The listing builds one solid part. Answer for the finished solid, in the listing's coordinates (mm). Face numbers are marked on the shaded views. A direction names the side the tool comes from. Round coordinates to 2 decimals unless told otherwise and drop trailing zeros. Order: outer loops, then holes, each group sorted by start corner. A loop starts at its lowest first (then second) coordinate and runs counter-clockwise, first axis right, second up. Notation, with made-up numbers: M 78.5,-38 L 122.5,-38 A19 cw 122.5,-3 Z; hole C -12,13 d2. An arc over 180 degrees is marked long. Put each result on its own line as item: value. Start each with the question number.
1. The part is cut by section B-B (z = 8). Give the vertices of the cut face in (x, y), then the cut area to 3 significant figures.
2. The part is cut by section C-C (z = 4.5). Give the vertices of the cut face in (x, y), then the cut area to 3 significant figures.
3. Which of the six approach directions +Z, -Z, +X, -X, +Y, -Y give full straight-line access (tool end or side, diameter ignored) to the marked faces 1 and 2?
4. Consider line 1 (Z direction, x = -0.7, y = 10); line 2 (X direction, y = 5, z = -7.75); line 3 (Y direction, x = 41, z = -1.5). Determine where each line is inside the solid, lowest interval first.
5. Each of these flat-tipped pins is pushed along its axis until it touches: pin 1 Ø1 at (x, z) = (41, 11.5) entering from +Y; pin 2 Ø12 at (x, z) = (35, 0) entering from -Y; pin 3 Ø3 at (x, z) = (38, -10) entering from +Y. Where does it stop, or does it pass through?
6. The part is cut by section A-A (y = 11.5). Give the vertices of the cut face in (x, z).
7. The part is cut by section D-D (x = 47.5). Give the vertices of the cut face in (y, z).
from build123d import *

# Parameters (mm, degrees)
SM_BASE_FLANGE_1_DEPTH = 15
SKETCH_6_R             = 2.5
CUT_EXTRUDE_664_DEPTH  = 10
SKETCH_7_R             = 6.5
CUT_EXTRUDE_2_DEPTH    = 10


# Sheet-metal steps are written as plain solids
with BuildPart() as part:
    # Sketch 1 → Базовая кромка1 (new, symmetric)
    with BuildSketch(Plane.XY):
        with BuildLine():
            Line((0, 20), (0, 1.089813792))
            ThreePointArc((0, 1.089813792), (0.286474508, 0.208135914), (1.036474508, -0.336770982))
            Line((1.036474508, -0.336770982), (52.308108396, -16.995934691))
            Line((52.308108396, -16.995934691), (51.844582905, -18.422519465))
            Line((51.844582905, -18.422519465), (0.572949017, -1.763355757))
            ThreePointArc((0.572949017, -1.763355757), (-0.927050983, -0.673541965), (-1.5, 1.089813792))
            Line((-1.5, 1.089813792), (-1.5, 20))
            Line((-1.5, 20), (0, 20))
        make_face()
    extrude(amount=SM_BASE_FLANGE_1_DEPTH, both=True)

    # Эскиз6 → Cut-Extrude 664 (cut)
    with BuildSketch(Plane(origin=(0, 0, 0), x_dir=(0, 0, -1), z_dir=(1, 0, 0))):
        with Locations(Location((-8, 10, 0), (0, 0, 90))):
            Circle(SKETCH_6_R)
        with Locations(Location((8, 10, 0), (0, 0, 90))):
            Circle(SKETCH_6_R)
    extrude(amount=-CUT_EXTRUDE_664_DEPTH, mode=Mode.SUBTRACT)

    # Эскиз7 → Вырез-Вытянуть2 (cut)
    with BuildSketch(Plane(origin=(0, 0, 0), x_dir=(0.9510565162951546, -0.3090169943749447, 0), z_dir=(0.3090169943749447, 0.9510565162951546, 0))):
        with Locations(Location((30, 0, 0), (0, 0, 180))):
            Circle(SKETCH_7_R)
    extrude(amount=-CUT_EXTRUDE_2_DEPTH, mode=Mode.SUBTRACT)


solid = part.part
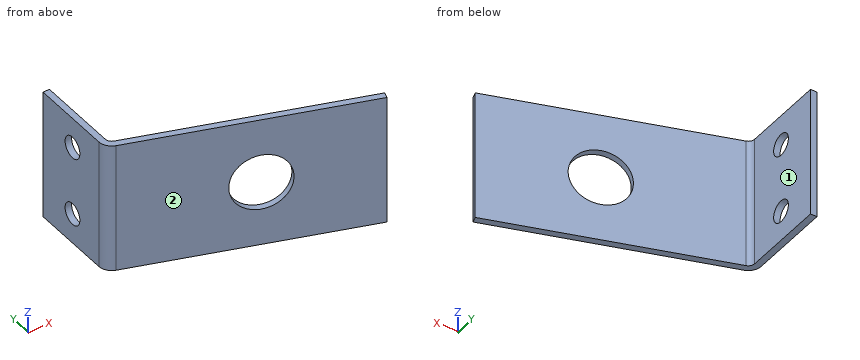
Resolved:
1. outline: M -1.5,1.09 A3 ccw 0.57,-1.76 L 51.84,-18.42 L 52.31,-17 L 1.04,-0.34 A1.5 cw 0,1.09 L 0,7.5 L -1.5,7.5 Z; M -1.5,12.5 L 0,12.5 L 0,20 L -1.5,20 Z
1. area: 106 mm2
2. outline: M -1.5,1.09 A3 ccw 0.57,-1.76 L 23.61,-9.25 L 24.07,-7.82 L 1.04,-0.34 A1.5 cw 0,1.09 L 0,20 L -1.5,20 Z; M 32.53,-12.15 L 51.84,-18.42 L 52.31,-17 L 32.99,-10.72 Z
2. area: 99.4 mm2
3. face 1: +Z, -Z, +X, +Y
3. face 2: +Z, -Z, -X, -Y
4. line 1: -15 to -10.5, -5.5 to 5.5, 10.5 to 15
4. line 2: -1.5 to 0
4. line 3: -14.9 to -13.32
5. pin 1: y = -13.16
5. pin 2: y = -14.9
5. pin 3: y = -11.86
6. outline: M -1.5,-15 L 0,-15 L 0,-10 L -1.5,-10 Z; M -1.5,-6 L 0,-6 L 0,6 L -1.5,6 Z; M -1.5,10 L 0,10 L 0,15 L -1.5,15 Z
7. outline: M -17.01,-15 L -15.43,-15 L -15.43,15 L -17.01,15 Z
